Build history of the part. All positions in model axes, mm. Give positions to 0.01 mm unless a question says otherwise; leave off trailing zeros. Order: outer loops, then holes, each group sorted by start corner. A loop starts at its lowest first (then second) coordinate and runs counter-clockwise, first axis right, second up. Notation, with made-up numbers: (35.5, -21.75) -> (75.5, -21.75) arc R19 cw to (75.5, -0.75) -> close; hole circle Ø2 at (-10.75, 41). An arc over 180 degrees is marked (long way). One line per item, written item: value. Start each with the question number.
(1) Probe line 1 (X direction, y = 0.9, z = 13.5); line 2 (X direction, y = 1.15, z = 29.25); line 3 (Z direction, x = 61.5, y = 1.15) (3 decimals). List the from-to ranges inside material, lowest first.
(2) Saw through at D-D on x = 74.5. Give the cut face in (y, z) (3 decimals).
(3) Saw through at B-B on x = 26.5. Give the cut face in (y, z) (3 decimals).
(4) Pin check, flat tips, straight feed: pin 1 (1 mm diameter, centred on x = 76, y = 1, fed in from +Z) (3 decimals); pin 2 (1 mm diameter, centred on y = 1.5, z = 29, fed in from -X); pin 3 (1 mm diameter, centred on y = 2.5, z = 24, fed in from +X) (3 decimals). Stop position of each tip, or through.
(5) Saw through at C-C on y = 1.25. Count the separate pieces of the cut face and the enclosed holes in it, plus the area to 3 significant figures.
(6) Saw through at A-A on z = 27.75. Give the cut face in (x, y) (3 decimals), plus the area to 3 significant figures.
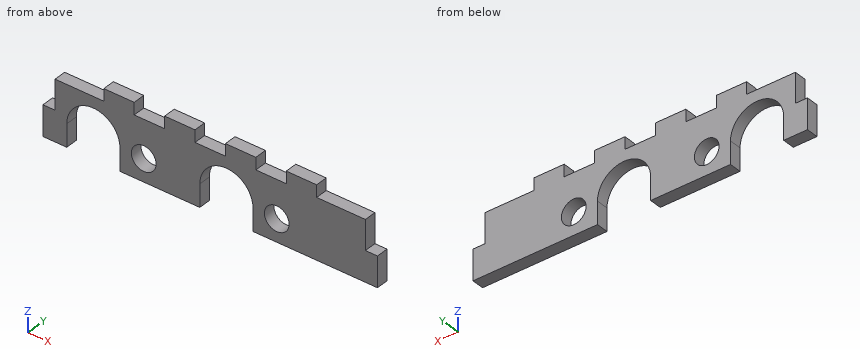
```python
from build123d import *

# Parameters (mm, degrees)
SKETCH3_W           = 88
SKETCH3_H           = 30
BOSS_EXTRUDE1_DEPTH = 3.175
CUT_EXTRUDE1_REACH  = 5.175
SKETCH4_W           = 3.175
SKETCH4_H           = 7.825
SKETCH4_W_2         = 8
SKETCH4_H_2         = 3.175
SKETCH4_H_3         = 11
CUT_EXTRUDE2_REACH  = 5.175
SKETCH5_R           = 3.25
CUT_EXTRUDE3_REACH  = 5.175
SKETCH6_W           = 81.65
SKETCH6_H           = 11
CUT_EXTRUDE4_REACH  = 5.175


with BuildPart() as part:
    # Sketch3 → Boss-Extrude1 (new body)
    with BuildSketch(Plane(origin=(0, 0, 0), x_dir=(1, 0, 0), z_dir=(0, 1, 0))):
        with Locations((44, -15)):
            Rectangle(SKETCH3_W, SKETCH3_H)
    extrude(amount=BOSS_EXTRUDE1_DEPTH)

    # Sketch4 → Cut-Extrude1 (cut, up to next)
    with BuildSketch(Plane(origin=(0, 3.175, 0), x_dir=(1, 0, 0), z_dir=(0, 1, 0)), mode=Mode.PRIVATE) as cut_extrude1_sk1:
        with Locations((1.5875, -22.9125)):
            Rectangle(SKETCH4_W, SKETCH4_H)
    cut_extrude1_tool1 = extrude(cut_extrude1_sk1.sketch, amount=-CUT_EXTRUDE1_REACH, mode=Mode.PRIVATE) & part.part
    add(cut_extrude1_tool1.solids().sort_by_distance((1.5875, 3.175, 22.9125))[0], mode=Mode.SUBTRACT)
    # Sketch4 → Cut-Extrude1 (cut, up to next)
    with BuildSketch(Plane(origin=(0, 3.175, 0), x_dir=(1, 0, 0), z_dir=(0, 1, 0)), mode=Mode.PRIVATE) as cut_extrude1_sk2:
        Polygon((0, -30), (16, -30), (16, -26.825), (3.175, -26.825), (0, -26.825), align=None)
    cut_extrude1_tool2 = extrude(cut_extrude1_sk2.sketch, amount=-CUT_EXTRUDE1_REACH, mode=Mode.PRIVATE) & part.part
    add(cut_extrude1_tool2.solids().sort_by_distance((8, 3.175, 28.4125))[0], mode=Mode.SUBTRACT)
    # Sketch4 → Cut-Extrude1 (cut, up to next)
    with BuildSketch(Plane(origin=(0, 3.175, 0), x_dir=(1, 0, 0), z_dir=(0, 1, 0)), mode=Mode.PRIVATE) as cut_extrude1_sk3:
        with Locations((28, -28.4125)):
            Rectangle(SKETCH4_W_2, SKETCH4_H_2)
    cut_extrude1_tool3 = extrude(cut_extrude1_sk3.sketch, amount=-CUT_EXTRUDE1_REACH, mode=Mode.PRIVATE) & part.part
    add(cut_extrude1_tool3.solids().sort_by_distance((28, 3.175, 28.4125))[0], mode=Mode.SUBTRACT)
    # Sketch4 → Cut-Extrude1 (cut, up to next)
    with BuildSketch(Plane(origin=(0, 3.175, 0), x_dir=(1, 0, 0), z_dir=(0, 1, 0)), mode=Mode.PRIVATE) as cut_extrude1_sk4:
        with Locations((44, -28.4125)):
            Rectangle(SKETCH4_W_2, SKETCH4_H_2)
    cut_extrude1_tool4 = extrude(cut_extrude1_sk4.sketch, amount=-CUT_EXTRUDE1_REACH, mode=Mode.PRIVATE) & part.part
    add(cut_extrude1_tool4.solids().sort_by_distance((44, 3.175, 28.4125))[0], mode=Mode.SUBTRACT)
    # Sketch4 → Cut-Extrude1 (cut, up to next)
    with BuildSketch(Plane(origin=(0, 3.175, 0), x_dir=(1, 0, 0), z_dir=(0, 1, 0)), mode=Mode.PRIVATE) as cut_extrude1_sk5:
        with Locations((60, -28.4125)):
            Rectangle(SKETCH4_W_2, SKETCH4_H_2)
    cut_extrude1_tool5 = extrude(cut_extrude1_sk5.sketch, amount=-CUT_EXTRUDE1_REACH, mode=Mode.PRIVATE) & part.part
    add(cut_extrude1_tool5.solids().sort_by_distance((60, 3.175, 28.4125))[0], mode=Mode.SUBTRACT)
    # Sketch4 → Cut-Extrude1 (cut, up to next)
    with BuildSketch(Plane(origin=(0, 3.175, 0), x_dir=(1, 0, 0), z_dir=(0, 1, 0)), mode=Mode.PRIVATE) as cut_extrude1_sk6:
        with Locations((86.4125, -22.9125)):
            Rectangle(SKETCH4_W, SKETCH4_H)
    cut_extrude1_tool6 = extrude(cut_extrude1_sk6.sketch, amount=-CUT_EXTRUDE1_REACH, mode=Mode.PRIVATE) & part.part
    add(cut_extrude1_tool6.solids().sort_by_distance((86.4125, 3.175, 22.9125))[0], mode=Mode.SUBTRACT)
    # Sketch4 → Cut-Extrude1 (cut, up to next)
    with BuildSketch(Plane(origin=(0, 3.175, 0), x_dir=(1, 0, 0), z_dir=(0, 1, 0)), mode=Mode.PRIVATE) as cut_extrude1_sk7:
        with Locations((86.4125, -5.5)):
            Rectangle(SKETCH4_W, SKETCH4_H_3)
    cut_extrude1_tool7 = extrude(cut_extrude1_sk7.sketch, amount=-CUT_EXTRUDE1_REACH, mode=Mode.PRIVATE) & part.part
    add(cut_extrude1_tool7.solids().sort_by_distance((86.4125, 3.175, 5.5))[0], mode=Mode.SUBTRACT)
    # Sketch4 → Cut-Extrude1 (cut, up to next)
    with BuildSketch(Plane(origin=(0, 3.175, 0), x_dir=(1, 0, 0), z_dir=(0, 1, 0)), mode=Mode.PRIVATE) as cut_extrude1_sk8:
        Polygon((72, -26.825), (72, -30), (88, -30), (88, -26.825), (84.825, -26.825), align=None)
    cut_extrude1_tool8 = extrude(cut_extrude1_sk8.sketch, amount=-CUT_EXTRUDE1_REACH, mode=Mode.PRIVATE) & part.part
    add(cut_extrude1_tool8.solids().sort_by_distance((80, 3.175, 28.4125))[0], mode=Mode.SUBTRACT)
    # Sketch4 → Cut-Extrude1 (cut, up to next)
    with BuildSketch(Plane(origin=(0, 3.175, 0), x_dir=(1, 0, 0), z_dir=(0, 1, 0)), mode=Mode.PRIVATE) as cut_extrude1_sk9:
        with Locations((1.5875, -5.5)):
            Rectangle(SKETCH4_W, SKETCH4_H_3)
    cut_extrude1_tool9 = extrude(cut_extrude1_sk9.sketch, amount=-CUT_EXTRUDE1_REACH, mode=Mode.PRIVATE) & part.part
    add(cut_extrude1_tool9.solids().sort_by_distance((1.5875, 3.175, 5.5))[0], mode=Mode.SUBTRACT)

    # Sketch5 → Cut-Extrude2 (cut, up to next)
    with BuildSketch(Plane(origin=(0, 3.175, 0), x_dir=(1, 0, 0), z_dir=(0, 1, 0)), mode=Mode.PRIVATE) as cut_extrude2_sk1:
        with Locations((61.5, -16.915)):
            Circle(SKETCH5_R)
    cut_extrude2_tool1 = extrude(cut_extrude2_sk1.sketch, amount=-CUT_EXTRUDE2_REACH, mode=Mode.PRIVATE) & part.part
    add(cut_extrude2_tool1.solids().sort_by_distance((61.5, 3.175, 16.915))[0], mode=Mode.SUBTRACT)
    # Sketch5 → Cut-Extrude2 (cut, up to next)
    with BuildSketch(Plane(origin=(0, 3.175, 0), x_dir=(1, 0, 0), z_dir=(0, 1, 0)), mode=Mode.PRIVATE) as cut_extrude2_sk2:
        with Locations((26.5, -16.915)):
            Circle(SKETCH5_R)
    cut_extrude2_tool2 = extrude(cut_extrude2_sk2.sketch, amount=-CUT_EXTRUDE2_REACH, mode=Mode.PRIVATE) & part.part
    add(cut_extrude2_tool2.solids().sort_by_distance((26.5, 3.175, 16.915))[0], mode=Mode.SUBTRACT)

    # Sketch6 → Cut-Extrude3 (cut, up to next)
    with BuildSketch(Plane(origin=(0, 3.175, 0), x_dir=(1, 0, 0), z_dir=(0, 1, 0)), mode=Mode.PRIVATE) as cut_extrude3_sk1:
        with Locations((44, -5.5)):
            Rectangle(SKETCH6_W, SKETCH6_H)
    cut_extrude3_tool1 = extrude(cut_extrude3_sk1.sketch, amount=-CUT_EXTRUDE3_REACH, mode=Mode.PRIVATE) & part.part
    add(cut_extrude3_tool1.solids().sort_by_distance((44, 3.175, 5.5))[0], mode=Mode.SUBTRACT)

    # Sketch7 → Cut-Extrude4 (cut, up to next)
    with BuildSketch(Plane(origin=(0, 3.175, 0), x_dir=(1, 0, 0), z_dir=(0, 1, 0)), mode=Mode.PRIVATE) as cut_extrude4_sk1:
        with BuildLine():
            Line((6.25, -16.915), (6.25, -11))
            Line((6.25, -11), (20.25, -11))
            Line((20.25, -11), (20.25, -16.915))
            ThreePointArc((20.25, -16.915), (13.25, -23.915), (6.25, -16.915))
        make_face()
    cut_extrude4_tool1 = extrude(cut_extrude4_sk1.sketch, amount=-CUT_EXTRUDE4_REACH, mode=Mode.PRIVATE) & part.part
    add(cut_extrude4_tool1.solids().sort_by_distance((13.25, 3.175, 16.813335))[0], mode=Mode.SUBTRACT)
    # Sketch7 → Cut-Extrude4 (cut, up to next)
    with BuildSketch(Plane(origin=(0, 3.175, 0), x_dir=(1, 0, 0), z_dir=(0, 1, 0)), mode=Mode.PRIVATE) as cut_extrude4_sk2:
        with BuildLine():
            Line((41.25, -16.915), (41.25, -11))
            Line((41.25, -11), (55.25, -11))
            Line((55.25, -11), (55.25, -16.915))
            ThreePointArc((55.25, -16.915), (48.25, -23.915), (41.25, -16.915))
        make_face()
    cut_extrude4_tool2 = extrude(cut_extrude4_sk2.sketch, amount=-CUT_EXTRUDE4_REACH, mode=Mode.PRIVATE) & part.part
    add(cut_extrude4_tool2.solids().sort_by_distance((48.25, 3.175, 16.813335))[0], mode=Mode.SUBTRACT)


solid = part.part
```
Results below:
1. line 1: x = 0 to 6.25, 20.25 to 41.25, 55.25 to 88
1. line 2: x = 16 to 24, 32 to 40, 48 to 56, 64 to 72
1. line 3: z = 11 to 13.665, 20.165 to 26.825
2. outline: (0, 11) -> (3.175, 11) -> (3.175, 26.825) -> (0, 26.825) -> close
3. outline: (0, 11) -> (3.175, 11) -> (3.175, 13.665) -> (0, 13.665) -> close; (0, 20.165) -> (3.175, 20.165) -> (3.175, 26.825) -> (0, 26.825) -> close
4. pin 1: stops at z = 26.825
4. pin 2: stops at x = 16
4. pin 3: stops at x = 84.825
5. separate pieces: 1
5. enclosed holes: 2
5. area: 1,060 mm²
6. outline: (16, 0) -> (24, 0) -> (24, 3.175) -> (16, 3.175) -> close; (32, 0) -> (40, 0) -> (40, 3.175) -> (32, 3.175) -> close; (48, 0) -> (56, 0) -> (56, 3.175) -> (48, 3.175) -> close; (64, 0) -> (72, 0) -> (72, 3.175) -> (64, 3.175) -> close
6. area: 102 mm²
